```python
from build123d import *

# Parameters (mm, degrees)
F1_DEPTH = 20


with BuildPart() as f1:
    # F0 (on Top) → F1 (new body)
    with BuildSketch(Plane.XY):
        Polygon((-90.849426, 50), (-90.849426, 0), (0, 0), (90.849426, 0), (90.849426, 50), (85.849426, 50), (85.849426, 10), (75.849426, 10), (65.849426, 10), (65.849426, 70), (65.849426, 90), (65.849426, 100), (-65.849426, 100), (-65.849426, 90), (-65.849426, 70), (-65.849426, 10), (-75.849426, 10), (-85.849426, 10), (-85.849426, 50), (-85.849426, 70), (-90.849426, 70), align=None)
        with BuildLine():
            ThreePointArc((35, 50), (24.748737, 25.251263), (0, 15))
            ThreePointArc((0, 15), (-24.748737, 74.748737), (35, 50))
        make_face(mode=Mode.SUBTRACT)
    extrude(amount=F1_DEPTH)


solid = f1.part
```
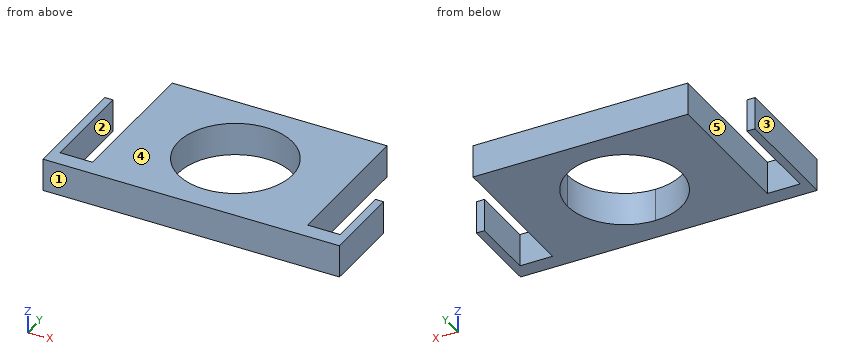
Geometry: final body of the model. Coordinates: model frame, mm. Face numbers are marked on the shaded views. A direction names the side the tool comes from. Round coordinates to 2 decimals unless told otherwise and drop trailing zeros. Order: outer loops, then holes, each group sorted by start corner. A loop starts at its lowest first (then second) coordinate and runs counter-clockwise, first axis right, second up. Notation, with made-up numbers: M 7.5,68 L 23.5,68 A23 cw 23.5,83 Z; hole C 29.5,-17 d11. An arc over 180 degrees is marked long. One line per item, written item: value.
(1) Cut plane D-D (y = 76). Return the cut outline in (x, z).
Result sheet:
outline: M -65.85,0 L -23.43,0 L -23.43,20 L -65.85,20 Z; M 23.43,0 L 65.85,0 L 65.85,20 L 23.43,20 Z
(2) Pull-direction query (X, two-part tool) for the marked faces 1, 2 and 3; classes: pulls with the +X half, pulls with the -X half, needs draft (parallel to the pull), parting line crosses it, or undercut.
Result sheet:
face 1: needs draft
face 2: undercut
face 3: pulls with the -X half
(3) Cut plane A-A (z = 14.5). Return the cut outline in (x, y).
Result sheet:
outline: M -90.85,0 L 90.85,0 L 90.85,50 L 85.85,50 L 85.85,10 L 65.85,10 L 65.85,100 L -65.85,100 L -65.85,10 L -85.85,10 L -85.85,70 L -90.85,70 Z; hole M 0,15 A35 ccw 35,50 A35 ccw long Z
(4) Line query: probe 1 along X at (y, z) = (49.5, 1.5); probe 2 along X at (y, z) = (42, 17.5); probe 3 along X at (y, z) = (63, 1.25). Output: solid intervals per line, ascending. Write a range as [from, to].
Result sheet:
probe 1: [-90.85, -85.85], [-65.85, -35], [35, 65.85], [85.85, 90.85]
probe 2: [-90.85, -85.85], [-65.85, -34.07], [34.07, 65.85], [85.85, 90.85]
probe 3: [-90.85, -85.85], [-65.85, -32.5], [32.5, 65.85]
(5) Cut plane C-C (x = 6.5). Return the cut outline in (y, z).
Result sheet:
outline: M 0,0 L 15.61,0 L 15.61,20 L 0,20 Z; M 84.39,0 L 100,0 L 100,20 L 84.39,20 Z
(6) Cut plane B-B (y = 45). Return the cut outline in (x, z).
Result sheet:
outline: M -90.85,0 L -85.85,0 L -85.85,20 L -90.85,20 Z; M -65.85,0 L -34.64,0 L -34.64,20 L -65.85,20 Z; M 34.64,0 L 65.85,0 L 65.85,20 L 34.64,20 Z; M 85.85,0 L 90.85,0 L 90.85,20 L 85.85,20 Z
(7) Pin query (flat end, axial travel): P1, Ø4, axis at x = -89, z = 8.5, coming from the +Y side; P2, Ø10, axis at x = 76.5, z = 6.5, coming from the +Y side; P3, Ø1.5, axis at x = 89.5, z = 15, coming from the +Y side. Return the tip coordinate at first contact, or that it passes through.
Result sheet:
P1: y = 70
P2: y = 10
P3: y = 50
(8) Reachability of the marked faces 4 and 5 from +Z, -Z, +X, -X, +Y, -Y: full face, straight path, thin tool, end or side. Return the list, or none.
Result sheet:
face 4: +Z, +X, -X, +Y, -Y
face 5: +Z, -Z, +Y
